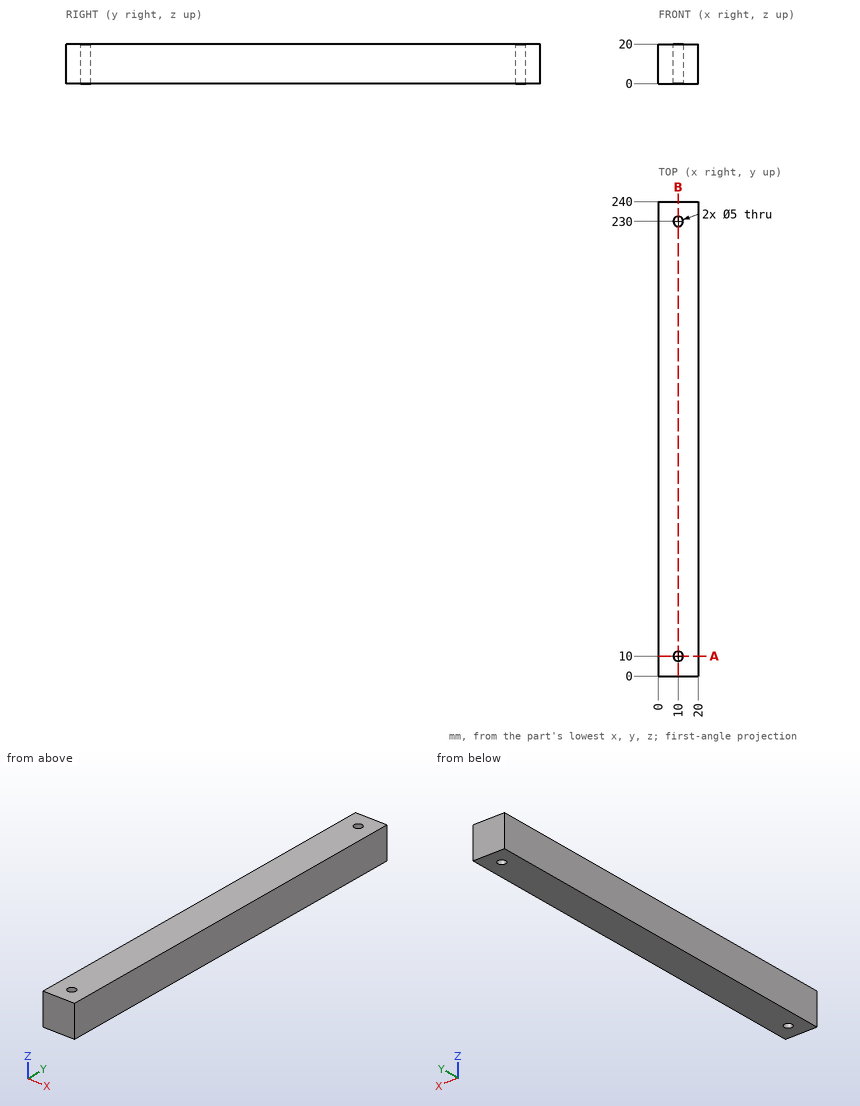
Could you check a few things on this drawing? It's one solid part, dimensions in mm from its lowest x, y, z. Round coordinates to 2 decimals unless told otherwise and drop trailing zeros. Order: outer loops, then holes, each group sorted by start corner. A loop starts at its lowest first (then second) coordinate and runs counter-clockwise, first axis right, second up. Notation, with made-up numbers: M 54.5,13.25 L 64.5,13.25 A35 ccw 64.5,51.25 Z; hole C 55,44.25 d3. An arc over 180 degrees is marked long. Use a Markdown table: item, result.
1) If I drill on line 1 along Y through (x, z) = (10, 8.25); line 2 along X through (y, z) = (230, 12.5); line 3 along Y through (x, z) = (10.5, 7.25), over which ranges is the centre line in solid material (lowest first)?
Geometry says:
| item | result |
|---|---|
| line 1 | y = 0 to 7.5, 12.5 to 227.5, 232.5 to 240 |
| line 2 | x = 0 to 7.5, 12.5 to 20 |
| line 3 | y = 0 to 7.55, 12.45 to 227.55, 232.45 to 240 |
2) Imagine slicing it at A-A (y = 10). List the corners of the cut face in (x, z) for me.
Geometry says:
| item | result |
|---|---|
| outline | M 0,0 L 7.5,0 L 7.5,20 L 0,20 Z; M 12.5,0 L 20,0 L 20,20 L 12.5,20 Z |
3) I'm going to push a flat-ended pin straight in: P1, Ø4, axis at x = 10, y = 10, coming from the +Z side. Where does the tip first touch, or does it pass through?
Geometry says:
| item | result |
|---|---|
| P1 | passes through |
4) Imagine slicing it at B-B (x = 10). List the corners of the cut face in (y, z) for me.
Geometry says:
| item | result |
|---|---|
| outline | M 0,0 L 7.5,0 L 7.5,20 L 0,20 Z; M 12.5,0 L 227.5,0 L 227.5,20 L 12.5,20 Z; M 232.5,0 L 240,0 L 240,20 L 232.5,20 Z |
